Read the model definition and answer for the solid it produces. Units are mm, in the model's axes. Face numbers are marked on the shaded views. A direction names the side the tool comes from. Coordinates: 2 decimals unless noted, no trailing zeros. Write each loop counter-clockwise with the first axis right and the second up, starting at its lowest first coordinate (ties: lowest second). Pieces come first, ordered by that corner, then holes. Notation, with made-up numbers: (25, -29) -> (32, -29) arc R17 cw to (32, 1) -> close; hole circle Ø8 at (10.25, 9). An arc over 180 degrees is marked (long way). Use CSV: the item, a comma, the result in double quotes.
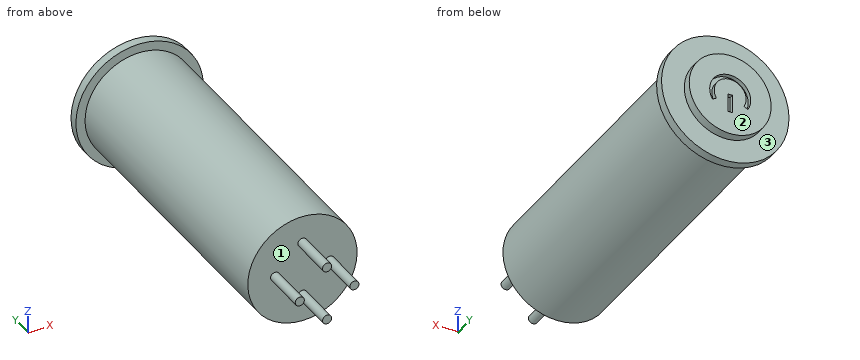
from build123d import *

# Parameters (mm, degrees)
SKETCH_1_R          = 7
EXTRUDE_1_DEPTH     = 1
SKETCH_2_R          = 4.5
EXTRUDE_2_DEPTH     = 1
SKETCH_3_W          = 0.5
SKETCH_3_H          = 2
CUT_EXTRUDE_1_DEPTH = 0.5
SKETCH_4_R          = 6
EXTRUDE_3_DEPTH     = 33
SKETCH_5_R          = 0.5
EXTRUDE_4_DEPTH     = 5


with BuildPart() as part:
    # 草图1 → 凸台-拉伸1 (new body)
    with BuildSketch(Plane(origin=(0, 0, 0), x_dir=(1, 0, 0), z_dir=(0, 1, 0))):
        with Locations(Location((0, 0, 0), (0, 0, 270))):
            Circle(SKETCH_1_R)
    extrude(amount=EXTRUDE_1_DEPTH)

    # 草图2 → 凸台-拉伸2 (add)
    with BuildSketch(Plane(origin=(0, 1, 0), x_dir=(1, 0, 0), z_dir=(0, 1, 0))):
        with Locations(Location((0, 0, 0), (0, 0, 270))):
            Circle(SKETCH_2_R)
    extrude(amount=EXTRUDE_2_DEPTH)

    # 草图3 → 切除-拉伸-薄壁1 (cut)
    with BuildSketch(Plane(origin=(0, 2, 0), x_dir=(1, 0, 0), z_dir=(0, 1, 0))):
        with Locations((0, 1)):
            Rectangle(SKETCH_3_W, SKETCH_3_H)
        with BuildLine():
            ThreePointArc((-1.948557159, 1.125), (0, -2.25), (1.948557159, 1.125))
            Line((1.948557159, 1.125), (1.515544457, 0.875))
            ThreePointArc((1.515544457, 0.875), (0, -1.75), (-1.515544457, 0.875))
            Line((-1.515544457, 0.875), (-1.948557159, 1.125))
        make_face()
    extrude(amount=-CUT_EXTRUDE_1_DEPTH, mode=Mode.SUBTRACT)

    # 草图4 → 凸台-拉伸3 (add)
    with BuildSketch(Plane.XZ):
        with Locations(Location((0, 0, 0), (0, 0, 270))):
            Circle(SKETCH_4_R)
    extrude(amount=EXTRUDE_3_DEPTH)

    # 草图5 → 凸台-拉伸4 (add)
    with BuildSketch(Plane.XZ.offset(33)):
        with Locations(Location((0, 3, 0), (0, 0, 270))):
            Circle(SKETCH_5_R)
        with Locations(Location((3, 0, 0), (0, 0, 270))):
            Circle(SKETCH_5_R)
        with Locations(Location((0, -3, 0), (0, 0, 270))):
            Circle(SKETCH_5_R)
        with Locations(Location((-3, 0, 0), (0, 0, 270))):
            Circle(SKETCH_5_R)
    extrude(amount=EXTRUDE_4_DEPTH)


solid = part.part
1. Find the intervals of material crossed by line 1 along Z through (x, y) = (-0.25, -9.5); line 2 along Y through (x, z) = (5.25, -1.75), in increasing order.
Solutions:
line 1,"z = -5.99 to 5.99"
line 2,"y = -33 to 1"
2. Each of these flat-tipped pins is pushed along its axis until it touches: pin 1 Ø5 at (x, z) = (5.5, 2) entering from +Y; pin 2 Ø8 at (y, z) = (-30, -0.5) entering from -X; pin 3 Ø8 at (x, y) = (3.5, -31.5) entering from +Z; pin 4 Ø3 at (y, z) = (-25.5, 2.5) entering from +X. Where does it stop, or does it pass through?
Solutions:
pin 1,"stops at y = 2"
pin 2,"stops at x = -6"
pin 3,"stops at z = 6"
pin 4,"stops at x = 5.92"
3. A cutting plane is placed at C-C (y = -7). Give the vertices of the cut face in (x, z), and give its area (3 significant figures).
Solutions:
outline,"circle Ø12 at (0, 0)"
area,"113 mm^2"
4. A tool of negligible diameter and unlimited length cuts with its end or side. For the marked faces 1, 2 and 3, from which of +Z, -Z, +X, -X, +Y, -Y can it reach the whole face along a straight path? Write none if from no direction.
Solutions:
face 1,"-Y"
face 2,"+Z, -Z, +X, -X, +Y"
face 3,"+Y"
5. A cutting plane is placed at B-B (x = 5.25). Give the vertices of the cut face in (y, z).
Solutions:
outline,"(-33, -2.9) -> (0, -2.9) -> (0, -4.63) -> (1, -4.63) -> (1, 4.63) -> (0, 4.63) -> (0, 2.9) -> (-33, 2.9) -> close"
6. A cutting plane is placed at D-D (x = -1). Give the vertices of the cut face in (y, z).
Solutions:
outline,"(-33, -5.92) -> (0, -5.92) -> (0, -6.93) -> (1, -6.93) -> (1, -4.39) -> (2, -4.39) -> (2, 1.44) -> (1.5, 1.44) -> (1.5, 2.02) -> (2, 2.02) -> (2, 4.39) -> (1, 4.39) -> (1, 6.93) -> (0, 6.93) -> (0, 5.92) -> (-33, 5.92) -> close"
7. A cutting plane is placed at A-A (z = 3). Give the vertices of the cut face in (x, y), and give its area (3 significant figures).
Solutions:
outline,"(-6.32, 0) -> (-5.2, 0) -> (-5.2, -33) -> (-0.5, -33) -> (-0.5, -38) -> (0.5, -38) -> (0.5, -33) -> (5.2, -33) -> (5.2, 0) -> (6.32, 0) -> (6.32, 1) -> (3.35, 1) -> (3.35, 2) -> (-3.35, 2) -> (-3.35, 1) -> (-6.32, 1) -> close"
area,"367 mm^2"
